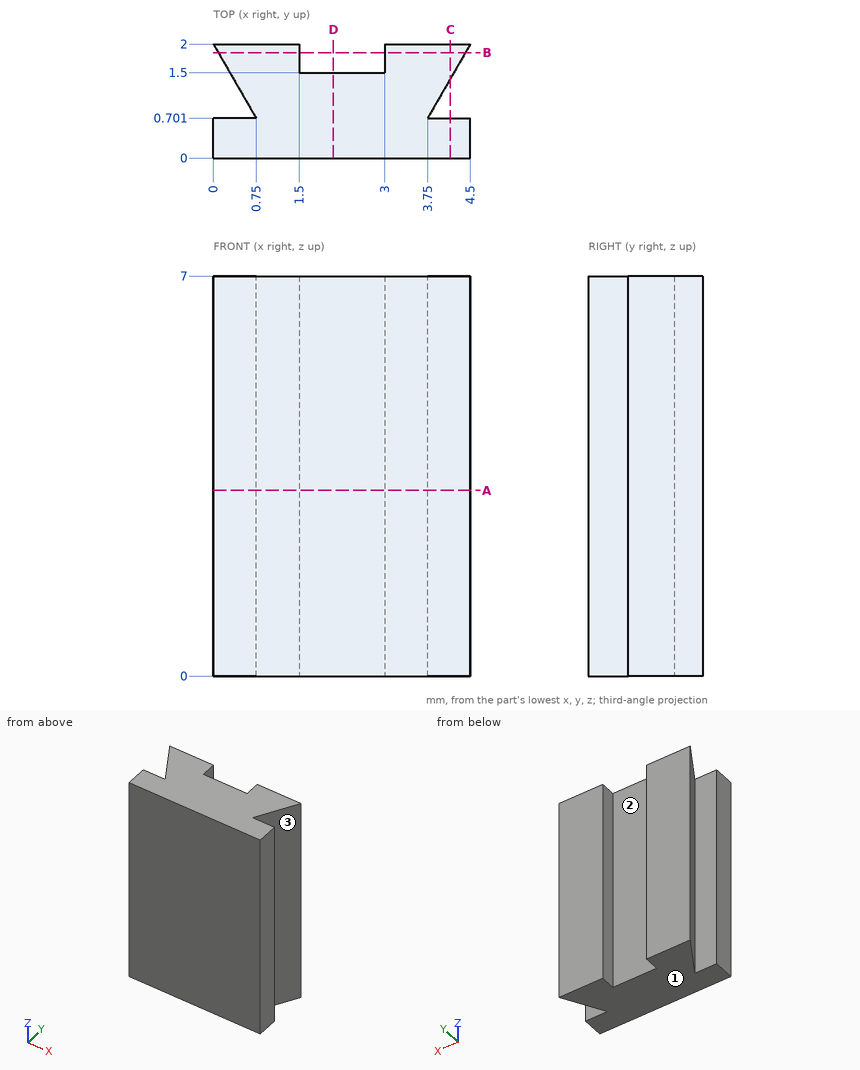
Input: dimensioned drawing with shaded views. Units: mm. Origin: part minimum x, y, z. Coordinates: 2 decimals unless noted, no trailing zeros. Loops run counter-clockwise (first coordinate to the right, second up) from the corner with the lowest first, then second, coordinate; pieces in that order, holes last. Notation, with made-up numbers: M 47,64 L 81,64 A11 ccw 81,71 Z; hole C 89,87.25 d9. An arc over 180 degrees is marked long. One line per item, written item: value. Start each with the question number.
1) Draft query along X for the marked faces 1, 2 and 3. Return one class per face: released by +X, released by -X, zero draft, split by the parting line, or undercut.
2) Cut plane B-B (y = 1.85). Return loops of the section in (x, z).
3) Pin query (flat end, axial travel): P1, Ø2, axis at x = 1.5, z = 1, coming from the -Y side. Return the tip coordinate at first contact, or that it passes through.
4) Material intervals for L1, parallel to Y at x = 2.5, z = 2.75; L2, parallel to X at y = 1.9, z = 4.75; L3, parallel to X at y = 1.65, z = 4, sorted ascending. Write a range as from..to.
5) Cut plane A-A (z = 3.25). Return loops of the section in (x, y).
6) Cut plane D-D (x = 2.1). Return loops of the section in (y, z), then the cut area to 3 significant figures.
7) Cut plane C-C (x = 4.15). Return loops of the section in (y, z).
Evaluation:
1. face 1: zero draft
1. face 2: undercut
1. face 3: released by +X
2. outline: M 0.09,0 L 1.5,0 L 1.5,7 L 0.09,7 Z; M 3,0 L 4.41,0 L 4.41,7 L 3,7 Z
3. P1: y = 0
4. L1: 0..1.5
4. L2: 0.06..1.5, 3..4.44
4. L3: 0.2..1.5, 3..4.3
5. outline: M 0,0 L 4.5,0 L 4.5,0.7 L 3.75,0.7 L 4.5,2 L 3,2 L 3,1.5 L 1.5,1.5 L 1.5,2 L 0,2 L 0.75,0.7 L 0,0.7 Z
6. outline: M 0,0 L 1.5,0 L 1.5,7 L 0,7 Z
6. area: 10.5 mm^2
7. outline: M 0,0 L 0.7,0 L 0.7,7 L 0,7 Z; M 1.39,0 L 2,0 L 2,7 L 1.39,7 Z
